```python
from build123d import *

# Parameters (mm, degrees)
EXTRUDE_1_DEPTH     = 45
CUT_EXTRUDE_1_REACH = 86.161
SKETCH_2_R          = 1.7
CUT_EXTRUDE_2_REACH = 83.939
SKETCH_3_R          = 1.7
SKETCH_3_R_2        = 1.5


with BuildPart() as part:
    # 草图1 → 凸台-拉伸1 (new body)
    with BuildSketch(Plane(origin=(0, 0, 0), x_dir=(1, 0, 0), z_dir=(0, 1, 0))):
        Polygon((0, 0), (30, 0), (30, 60), (33, 60), (33, -3), (0, -3), align=None)
    extrude(amount=EXTRUDE_1_DEPTH)

    # 草图2 → 切除-拉伸1 (cut, up to next)
    with BuildSketch(Plane.XY.offset(3), mode=Mode.PRIVATE) as cut_extrude_1_sk1:
        with Locations((3.5, 32.5)):
            Circle(SKETCH_2_R)
    cut_extrude_1_tool1 = extrude(cut_extrude_1_sk1.sketch, amount=-CUT_EXTRUDE_1_REACH, mode=Mode.PRIVATE) & part.part
    # 草图2 → 切除-拉伸1 (cut, up to next)
    with BuildSketch(Plane.XY.offset(3), mode=Mode.PRIVATE) as cut_extrude_1_sk2:
        with Locations((23.5, 32.5)):
            Circle(SKETCH_2_R)
    cut_extrude_1_tool2 = extrude(cut_extrude_1_sk2.sketch, amount=-CUT_EXTRUDE_1_REACH, mode=Mode.PRIVATE) & part.part
    # 草图2 → 切除-拉伸1 (cut, up to next)
    with BuildSketch(Plane.XY.offset(3), mode=Mode.PRIVATE) as cut_extrude_1_sk3:
        with Locations((23.5, 12.5)):
            Circle(SKETCH_2_R)
    cut_extrude_1_tool3 = extrude(cut_extrude_1_sk3.sketch, amount=-CUT_EXTRUDE_1_REACH, mode=Mode.PRIVATE) & part.part
    # 草图2 → 切除-拉伸1 (cut, up to next)
    with BuildSketch(Plane.XY.offset(3), mode=Mode.PRIVATE) as cut_extrude_1_sk4:
        with Locations((3.5, 12.5)):
            Circle(SKETCH_2_R)
    cut_extrude_1_tool4 = extrude(cut_extrude_1_sk4.sketch, amount=-CUT_EXTRUDE_1_REACH, mode=Mode.PRIVATE) & part.part
    add(cut_extrude_1_tool1.solids().sort_by_distance((3.5, 32.5, 3))[0], mode=Mode.SUBTRACT)
    add(cut_extrude_1_tool2.solids().sort_by_distance((23.5, 32.5, 3))[0], mode=Mode.SUBTRACT)
    add(cut_extrude_1_tool3.solids().sort_by_distance((23.5, 12.5, 3))[0], mode=Mode.SUBTRACT)
    add(cut_extrude_1_tool4.solids().sort_by_distance((3.5, 12.5, 3))[0], mode=Mode.SUBTRACT)

    # 草图3 → 切除-拉伸2 (cut, up to next)
    with BuildSketch(Plane(origin=(33, 0, 0), x_dir=(0, 0, -1), z_dir=(1, 0, 0)), mode=Mode.PRIVATE) as cut_extrude_2_sk1:
        with Locations((26, 6)):
            Circle(SKETCH_3_R)
    cut_extrude_2_tool1 = extrude(cut_extrude_2_sk1.sketch, amount=-CUT_EXTRUDE_2_REACH, mode=Mode.PRIVATE) & part.part
    # 草图3 → 切除-拉伸2 (cut, up to next)
    with BuildSketch(Plane(origin=(33, 0, 0), x_dir=(0, 0, -1), z_dir=(1, 0, 0)), mode=Mode.PRIVATE) as cut_extrude_2_sk2:
        with Locations((26, 39)):
            Circle(SKETCH_3_R)
    cut_extrude_2_tool2 = extrude(cut_extrude_2_sk2.sketch, amount=-CUT_EXTRUDE_2_REACH, mode=Mode.PRIVATE) & part.part
    # 草图3 → 切除-拉伸2 (cut, up to next)
    with BuildSketch(Plane(origin=(33, 0, 0), x_dir=(0, 0, -1), z_dir=(1, 0, 0)), mode=Mode.PRIVATE) as cut_extrude_2_sk3:
        with Locations((37, 15.25)):
            Circle(SKETCH_3_R)
    cut_extrude_2_tool3 = extrude(cut_extrude_2_sk3.sketch, amount=-CUT_EXTRUDE_2_REACH, mode=Mode.PRIVATE) & part.part
    # 草图3 → 切除-拉伸2 (cut, up to next)
    with BuildSketch(Plane(origin=(33, 0, 0), x_dir=(0, 0, -1), z_dir=(1, 0, 0)), mode=Mode.PRIVATE) as cut_extrude_2_sk4:
        with Locations((37, 29.75)):
            Circle(SKETCH_3_R)
    cut_extrude_2_tool4 = extrude(cut_extrude_2_sk4.sketch, amount=-CUT_EXTRUDE_2_REACH, mode=Mode.PRIVATE) & part.part
    # 草图3 → 切除-拉伸2 (cut, up to next)
    with BuildSketch(Plane(origin=(33, 0, 0), x_dir=(0, 0, -1), z_dir=(1, 0, 0)), mode=Mode.PRIVATE) as cut_extrude_2_sk5:
        with Locations((44.5, 39)):
            Circle(SKETCH_3_R_2)
    cut_extrude_2_tool5 = extrude(cut_extrude_2_sk5.sketch, amount=-CUT_EXTRUDE_2_REACH, mode=Mode.PRIVATE) & part.part
    # 草图3 → 切除-拉伸2 (cut, up to next)
    with BuildSketch(Plane(origin=(33, 0, 0), x_dir=(0, 0, -1), z_dir=(1, 0, 0)), mode=Mode.PRIVATE) as cut_extrude_2_sk6:
        with Locations((47.6, 6)):
            Circle(SKETCH_3_R_2)
    cut_extrude_2_tool6 = extrude(cut_extrude_2_sk6.sketch, amount=-CUT_EXTRUDE_2_REACH, mode=Mode.PRIVATE) & part.part
    # 草图3 → 切除-拉伸2 (cut, up to next)
    with BuildSketch(Plane(origin=(33, 0, 0), x_dir=(0, 0, -1), z_dir=(1, 0, 0)), mode=Mode.PRIVATE) as cut_extrude_2_sk7:
        with Locations((47.6, 39)):
            Circle(SKETCH_3_R_2)
    cut_extrude_2_tool7 = extrude(cut_extrude_2_sk7.sketch, amount=-CUT_EXTRUDE_2_REACH, mode=Mode.PRIVATE) & part.part
    # 草图3 → 切除-拉伸2 (cut, up to next)
    with BuildSketch(Plane(origin=(33, 0, 0), x_dir=(0, 0, -1), z_dir=(1, 0, 0)), mode=Mode.PRIVATE) as cut_extrude_2_sk8:
        with Locations((44.5, 6)):
            Circle(SKETCH_3_R_2)
    cut_extrude_2_tool8 = extrude(cut_extrude_2_sk8.sketch, amount=-CUT_EXTRUDE_2_REACH, mode=Mode.PRIVATE) & part.part
    add(cut_extrude_2_tool1.solids().sort_by_distance((33, 6, -26))[0], mode=Mode.SUBTRACT)
    add(cut_extrude_2_tool2.solids().sort_by_distance((33, 39, -26))[0], mode=Mode.SUBTRACT)
    add(cut_extrude_2_tool3.solids().sort_by_distance((33, 15.25, -37))[0], mode=Mode.SUBTRACT)
    add(cut_extrude_2_tool4.solids().sort_by_distance((33, 29.75, -37))[0], mode=Mode.SUBTRACT)
    add(cut_extrude_2_tool5.solids().sort_by_distance((33, 39, -44.5))[0], mode=Mode.SUBTRACT)
    add(cut_extrude_2_tool6.solids().sort_by_distance((33, 6, -47.6))[0], mode=Mode.SUBTRACT)
    add(cut_extrude_2_tool7.solids().sort_by_distance((33, 39, -47.6))[0], mode=Mode.SUBTRACT)
    add(cut_extrude_2_tool8.solids().sort_by_distance((33, 6, -44.5))[0], mode=Mode.SUBTRACT)


solid = part.part
```
Here's how the part is built. I have some questions about the finished solid (model axes, mm). A direction names the side the tool comes from. Coordinates: 2 decimals unless noted, no trailing zeros. Loops run counter-clockwise (first coordinate to the right, second up) from the corner with the lowest first, then second, coordinate; pieces in that order, holes last. Notation, with made-up numbers: M -39.5,-13 L -23.5,-13 A15 ccw -23.5,14 Z; hole C 37.5,-7.5 d8. An arc over 180 degrees is marked long. One line per item, written item: value.
1. On a 3-axis mill with a long thin cutter (end or side, diameter ignored), from which of +Z, -Z, +X, -X, +Y, -Y can I reach the whole of each face in a straight line? I mean faces 5 (the flat face through (30, 22, -30)), 6 (the cylindrical face through (31.5, 38.1, -43.3)). Say none if no direction works.
Geometry says:
face 5: -Z, -X, +Y, -Y
face 6: +X, -X
2. Imagine slicing it at B-B (y = 29.75). List the corners of the cut face in (x, z) for me.
Geometry says:
outline: M 0,0 L 30,0 L 30,-35.3 L 33,-35.3 L 33,3 L 0,3 Z; M 30,-60 L 33,-60 L 33,-38.7 L 30,-38.7 Z
3. Imagine slicing it at C-C (y = 39). List the corners of the cut face in (x, z) for me.
Geometry says:
outline: M 0,0 L 30,0 L 30,-24.3 L 33,-24.3 L 33,3 L 0,3 Z; M 30,-60 L 33,-60 L 33,-49.1 L 30,-49.1 Z; M 30,-46.1 L 33,-46.1 L 33,-46 L 30,-46 Z; M 30,-43 L 33,-43 L 33,-27.7 L 30,-27.7 Z
4. Thinking about a two-plate mould opening in Z: for faces 1 (the cylindrical face through (32, 6, -43)), 2 (the cylindrical face through (31.5, 4.5, -26.8)), 3 (the flat face through (17, 22, 3)), 4 (the cylindrical face through (24.3, 31, 1.5)), which applies, +Z half, -Z half, draft (parallel to the pull), parting line (faces both ways), or undercut?
Geometry says:
face 1: undercut
face 2: undercut
face 3: +Z half
face 4: draft
5. Imagine slicing it at A-A (x = 3.5). List the corners of the cut face in (y, z) for me, and give its area (3 significant figures).
Geometry says:
outline: M 0,0 L 10.8,0 L 10.8,3 L 0,3 Z; M 14.2,0 L 30.8,0 L 30.8,3 L 14.2,3 Z; M 34.2,0 L 45,0 L 45,3 L 34.2,3 Z
area: 115 mm2
6. Imagine slicing it at D-D (z = -44.5). List the corners of the cut face in (x, y) for me, and give its area (3 significant figures).
Geometry says:
outline: M 30,0 L 33,0 L 33,4.5 L 30,4.5 Z; M 30,7.5 L 33,7.5 L 33,37.5 L 30,37.5 Z; M 30,40.5 L 33,40.5 L 33,45 L 30,45 Z
area: 117 mm2
7. Will these pins go through, and if not, where does the flat tip stop? pin 1 Ø2.5 at (y, z) = (29.75, -37) entering from +X; pin 2 Ø4 at (y, z) = (39, -44.5) entering from -X; pin 3 Ø5.5 at (y, z) = (6, -26) entering from +X; pin 4 Ø1 at (x, y) = (9, 11) entering from -Z.
Geometry says:
pin 1: passes through
pin 2: stops at x = 30
pin 3: stops at x = 33
pin 4: stops at z = 0
8. Please list where these lines run through material, in increasing order: probe 1 along Y at (x, z) = (30.9, -47.6); probe 2 along Y at (x, z) = (31.05, -37); probe 3 along X at (y, z) = (6, -18.5).
Geometry says:
probe 1: y = 0 to 4.5, 7.5 to 37.5, 40.5 to 45
probe 2: y = 0 to 13.55, 16.95 to 28.05, 31.45 to 45
probe 3: x = 30 to 33
